For this review, use the dimensioned drawing (mm, ordinates from the lowest corner) and the shaded views. A direction names the side the tool comes from. Coordinates: 2 decimals unless noted, no trailing zeros. Order: outer loops, then holes, each group sorted by start corner. A loop starts at its lowest first (then second) coordinate and runs counter-clockwise, first axis right, second up. Notation, with made-up numbers: (19.25, 50) -> (63.25, 50) arc R21 ccw to (63.25, 83) -> close; hole circle Ø7 at (86, 32). An arc over 180 degrees is marked (long way). Return JSON: item names as keys, results as strings. Group by question number.
Item 1: For line 1 along Z through (x, y) = (15.25, 15.3); line 2 along X through (y, z) = (14.9, 18.5); line 3 along Z through (x, y) = (7.25, 17.85), list the stretches that pass through material, from the lowest coordinate up.
Item 2: Insertion check: pin 1 (3 mm diameter, centred on x = 12, z = 22.5, fed in from -Y); pin 2 (1.5 mm diameter, centred on y = 6, z = 10, fed in from -X); pin 3 (4 mm diameter, centred on y = 14, z = 13, fed in from +X); pin 4 (2.5 mm diameter, centred on x = 31, y = 3, fed in from +Z). Each pin has a flat end and moves straight along its axis. Give the tip position at first contact, or say it passes through.
Item 3: Take a section at A-A (x = 7.25). Write out the cut boundary in (y, z).
Item 4: Draft analysis for pull direction Z (two halves, no side actions). For the marked faces 6, 7 and 8, state which applies: +Z half, -Z half, draft (parallel to the pull), parting line (faces both ways), or undercut.
Item 5: Take a section at B-B (z = 6.5). Write out the cut boundary in (x, y), then the cut area to 3 significant figures.
Item 6: Machinability: for the marked faces 1, 2, 3, 4 and 5, which of the approach directions +Z, -Z, +X, -X, +Y, -Y give a long, thin tool a straight path to every point of the face, cutting with its end or side? Answer none if there is none.
Item 7: Take a section at D-D (z = 18.5). Write out the cut boundary in (x, y), then the cut area to 3 significant figures.
Item 8: Take a section at C-C (y = 9.75). Write out the cut boundary in (x, z).
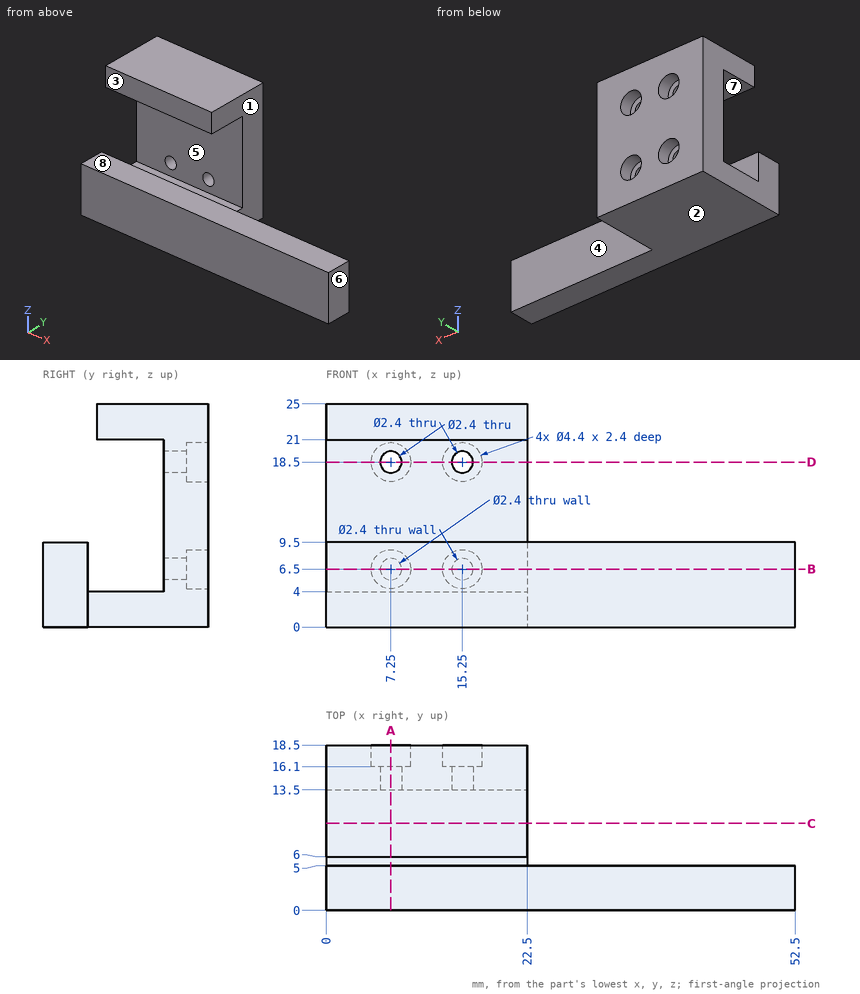
Findings below:
{
 "1": {"line 1": "z = 0 to 5.3, 7.7 to 17.3, 19.7 to 25", "line 2": "x = 0 to 6.05, 8.45 to 14.05, 16.45 to 22.5", "line 3": "z = 0 to 4.3, 8.7 to 16.3, 20.7 to 25"},
 "2": {"pin 1": "stops at y = 6", "pin 2": "passes through", "pin 3": "stops at x = 22.5", "pin 4": "stops at z = 9.5"},
 "3": {"outline": "(0, 0) -> (18.5, 0) -> (18.5, 4.3) -> (16.1, 4.3) -> (16.1, 5.3) -> (13.5, 5.3) -> (13.5, 4) -> (5, 4) -> (5, 9.5) -> (0, 9.5) -> close; (6, 21) -> (13.5, 21) -> (13.5, 19.7) -> (16.1, 19.7) -> (16.1, 20.7) -> (18.5, 20.7) -> (18.5, 25) -> (6, 25) -> close; (13.5, 7.7) -> (16.1, 7.7) -> (16.1, 8.7) -> (18.5, 8.7) -> (18.5, 16.3) -> (16.1, 16.3) -> (16.1, 17.3) -> (13.5, 17.3) -> close"},
 "4": {"face 6": "draft", "face 7": "undercut", "face 8": "+Z half"},
 "5": {"outline": "(0, 0) -> (52.5, 0) -> (52.5, 5) -> (0, 5) -> close; (0, 13.5) -> (6.05, 13.5) -> (6.05, 16.1) -> (5.05, 16.1) -> (5.05, 18.5) -> (0, 18.5) -> close; (8.45, 13.5) -> (14.05, 13.5) -> (14.05, 16.1) -> (13.05, 16.1) -> (13.05, 18.5) -> (9.45, 18.5) -> (9.45, 16.1) -> (8.45, 16.1) -> close; (16.45, 13.5) -> (22.5, 13.5) -> (22.5, 18.5) -> (17.45, 18.5) -> (17.45, 16.1) -> (16.45, 16.1) -> close", "area": "341 mm2"},
 "6": {"face 1": "+Z, -Z, +X, +Y", "face 2": "-Z, +X, -X, +Y, -Y", "face 3": "+Z, +X, -X, -Y", "face 4": "+Z, +X", "face 5": "+X, -X"},
 "7": {"outline": "(0, 13.5) -> (6.05, 13.5) -> (6.05, 16.1) -> (5.05, 16.1) -> (5.05, 18.5) -> (0, 18.5) -> close; (8.45, 13.5) -> (14.05, 13.5) -> (14.05, 16.1) -> (13.05, 16.1) -> (13.05, 18.5) -> (9.45, 18.5) -> (9.45, 16.1) -> (8.45, 16.1) -> close; (16.45, 13.5) -> (22.5, 13.5) -> (22.5, 18.5) -> (17.45, 18.5) -> (17.45, 16.1) -> (16.45, 16.1) -> close", "area": "78.9 mm2"},
 "8": {"outline": "(0, 0) -> (22.5, 0) -> (22.5, 4) -> (0, 4) -> close; (0, 21) -> (22.5, 21) -> (22.5, 25) -> (0, 25) -> close"}
}
